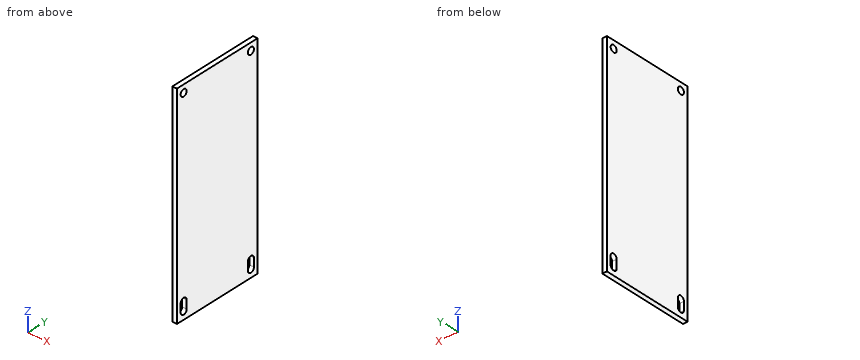
from build123d import *

# Parameters (mm, degrees)
SKETCH_1_W               = 139
SKETCH_1_H               = 60
EXTRUDE_1_DEPTH          = 1.5
HOLE_WIZARD_M4_1_D       = 4.5
HOLE_START               = -1.5
HOLE_WIZARD_M4_1_2_DEPTH = 3


# Read off the part's stored shape, not the designer's step: M4 间隙槽口1
with BuildPart() as part:
    # 草图1 → 凸台-拉伸1 (new, symmetric)
    with BuildSketch(Plane(origin=(0, 0, 0), x_dir=(0, 0, -1), z_dir=(1, 0, 0))):
        with Locations((69.5, 30)):
            Rectangle(SKETCH_1_W, SKETCH_1_H)
    extrude(amount=EXTRUDE_1_DEPTH, both=True)

    # Hole Wizard M4 _1 (through all)
    with Locations(Plane(origin=(1.5, 0, 0), x_dir=(0, 0, -1), z_dir=(1, 0, 0))):
        with Locations((5, 55), (5, 5)):
            Hole(HOLE_WIZARD_M4_1_D / 2)

    # Hole Wizard M4 _1 2 outline → Hole Wizard M4 _1 2 (cut)
    with BuildSketch(Plane.YZ.offset(HOLE_START)):
        with BuildLine():
            Line((7.25, -133.75), (7.25, -128.25))
            ThreePointArc((7.25, -128.25), (5, -126), (2.75, -128.25))
            Line((2.75, -128.25), (2.75, -133.75))
            ThreePointArc((2.75, -133.75), (5, -136), (7.25, -133.75))
        make_face()
        with BuildLine():
            Line((57.25, -133.75), (57.25, -128.25))
            ThreePointArc((57.25, -128.25), (55, -126), (52.75, -128.25))
            Line((52.75, -128.25), (52.75, -133.75))
            ThreePointArc((52.75, -133.75), (55, -136), (57.25, -133.75))
        make_face()
    extrude(amount=HOLE_WIZARD_M4_1_2_DEPTH, mode=Mode.SUBTRACT)


solid = part.part
Check sheet for the modelled part. Datum: model origin and axes. Units: mm. Coordinates: 2 decimals unless noted, no trailing zeros. Loops run counter-clockwise (first coordinate to the right, second up) from the corner with the lowest first, then second, coordinate; pieces in that order, holes last. Notation, with made-up numbers: (52.25, 55.25) -> (97.25, 55.25) arc R25 cw to (97.25, 77.25) -> close; hole circle Ø8 at (52, 11.25). An arc over 180 degrees is marked (long way). Answer in a Markdown table with one row per item.
1. Sectioned sample at B-B, the plane z = -5. Record the boundary of the cut face in (x, y).
Check values:
| item | result |
|---|---|
| outline | (-1.5, 0) -> (1.5, 0) -> (1.5, 2.75) -> (-1.5, 2.75) -> close; (-1.5, 7.25) -> (1.5, 7.25) -> (1.5, 52.75) -> (-1.5, 52.75) -> close; (-1.5, 57.25) -> (1.5, 57.25) -> (1.5, 60) -> (-1.5, 60) -> close |
2. Sectioned sample at A-A, the plane y = 55. Record the boundary of the cut face in (x, z), then the cut area to 4 significant figures.
Check values:
| item | result |
|---|---|
| outline | (-1.5, -139) -> (1.5, -139) -> (1.5, -136) -> (-1.5, -136) -> close; (-1.5, -126) -> (1.5, -126) -> (1.5, -7.25) -> (-1.5, -7.25) -> close; (-1.5, -2.75) -> (1.5, -2.75) -> (1.5, 0) -> (-1.5, 0) -> close |
| area | 373.5 mm2 |
3. Material ranges on line 1 along Y through (x, z) = (0.25, -5); line 2 along Z through (x, y) = (-1.2, 4); line 3 along Z through (x, y) = (0.05, 53), recorded low to high. Write a range as [from, to].
Check values:
| item | result |
|---|---|
| line 1 | y = [0, 2.75], [7.25, 52.75], [57.25, 60] |
| line 2 | z = [-139, -135.77], [-126.23, -7.02], [-2.98, 0] |
| line 3 | z = [-139, -134.78], [-127.22, -6.03], [-3.97, 0] |
4. Go/stop test with a flat-tipped pin: pin 1 (0.9 mm diameter, centred on x = 0.5, z = -131, fed in from -Y). Record where the tip stops, or that it passes through.
Check values:
| item | result |
|---|---|
| pin 1 | stops at y = 0 |
